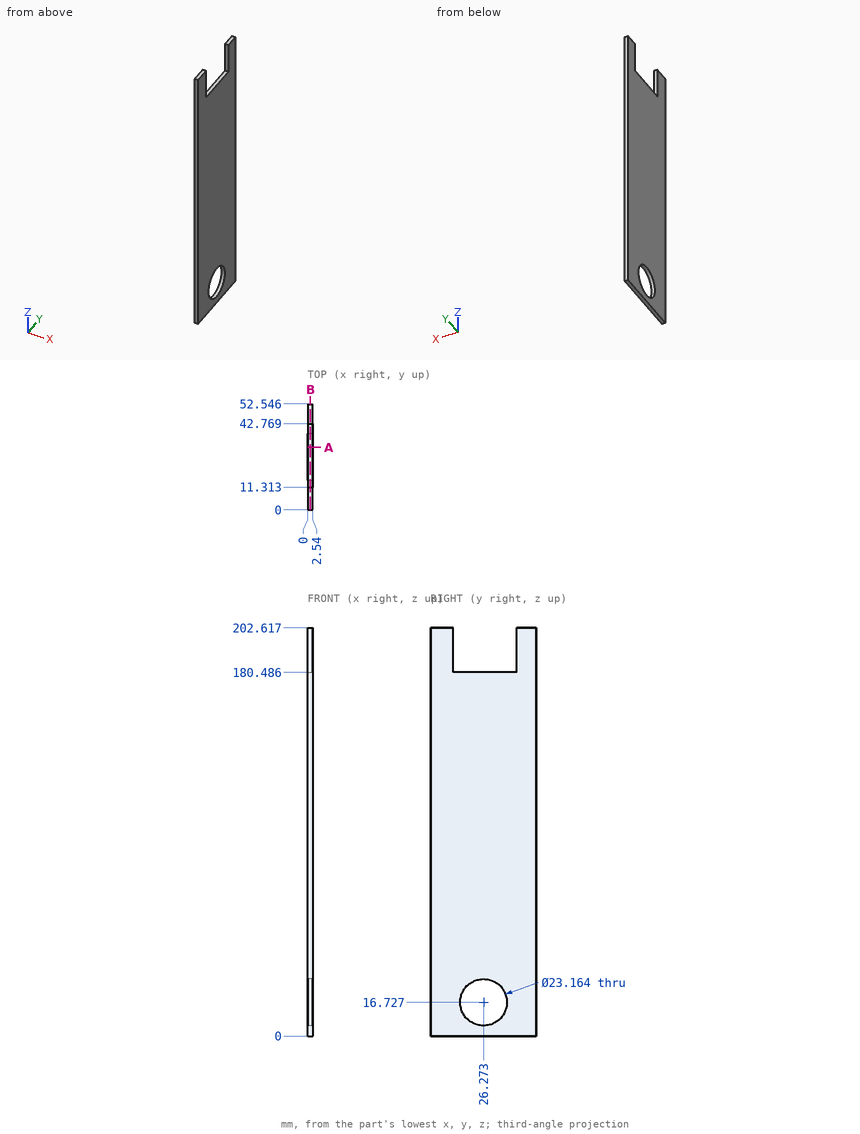
Verification items for this drawing (mm, ordinates from the low corner). Round coordinates to 2 decimals unless told otherwise and drop trailing zeros. Order: outer loops, then holes, each group sorted by start corner. A loop starts at its lowest first (then second) coordinate and runs counter-clockwise, first axis right, second up. Notation, with made-up numbers: (1.5, -35) - (52.5, -35) arc R22 ccw to (52.5, -10) - close; hole circle Ø2 at (34, 1.5). An arc over 180 degrees is marked (long way). Use CSV: the item, a comma, the result in double quotes.
(1) Section check A-A on y = 31. Record the boundary of the cut face in (x, z) (1 decimal).
Entries:
outline,"(0, 0) - (2.5, 0) - (2.5, 6.2) - (0, 6.2) - close; (0, 27.3) - (2.5, 27.3) - (2.5, 180.5) - (0, 180.5) - close"
(2) Thickness scan on probe 1 along Y at (x, z) = (1.5, 193.5); probe 2 along Y at (x, z) = (2.35, 25) (1 decimal); probe 3 along Z at (x, y) = (0.1, 23.5) (1 decimal). Record the ranges inside material, lowest first. Write a range as from..to.
Entries:
probe 1,"0..11.31, 42.77..52.55"
probe 2,"0..18.2, 34.4..52.5"
probe 3,"0..5.5, 28..180.5"
(3) Section check B-B on x = 1.45. Record the boundary of the cut face in (y, z) (1 decimal).
Entries:
outline,"(0, 0) - (52.5, 0) - (52.5, 202.6) - (42.8, 202.6) - (42.8, 180.5) - (11.3, 180.5) - (11.3, 202.6) - (0, 202.6) - close; hole circle Ø23.2 at (26.3, 16.7)"
(4) Gauge pin test, flat ends, axial feed: pin 1 Ø21 at (y, z) = (26.27, 16.73) entering from -X; pin 2 Ø0.8 at (x, y) = (0.5, 29.5) entering from +Z. Record the tip position at first contact, or that the pin passes through.
Entries:
pin 1,"through"
pin 2,"z = 180.49"
